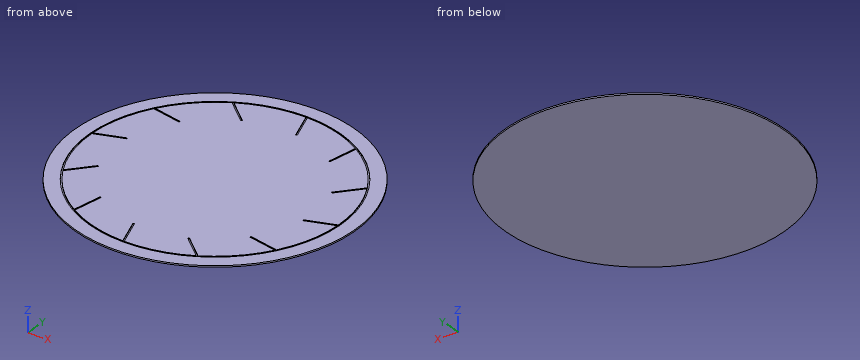
from build123d import *

# Parameters (mm, degrees)
SKETCH1_R           = 254
BOSS_EXTRUDE1_DEPTH = 2.54
SKETCH2_R           = 228.6
SKETCH2_R_2         = 226.06
CUT_EXTRUDE1_DEPTH  = 1.27
CUT_EXTRUDE2_DEPTH  = 1.27


with BuildPart() as part:
    # Sketch1 → Boss-Extrude1 (new body)
    with BuildSketch(Plane.XY):
        Circle(SKETCH1_R)
    extrude(amount=BOSS_EXTRUDE1_DEPTH)

    # Sketch2 → Cut-Extrude1 (cut)
    with BuildSketch(Plane.XY.offset(2.54)):
        Circle(SKETCH2_R)
        Circle(SKETCH2_R_2, mode=Mode.SUBTRACT)
    extrude(amount=-CUT_EXTRUDE1_DEPTH, mode=Mode.SUBTRACT)

    # Sketch4 → Cut-Extrude2 (cut)
    with BuildSketch(Plane.XY.offset(2.54)):
        with BuildLine():
            Line((-226.06, 0), (-175.26, 18.489687901))
            Line((-175.26, 18.489687901), (-176.128731164, 20.876507158))
            Line((-176.128731164, 20.876507158), (-226.043768674, 2.708919262))
            ThreePointArc((-226.043768674, 2.708919262), (-226.055942132, 1.354483944), (-226.06, 0))
        make_face()
        with BuildLine():
            Line((-195.77370278, 113.03), (-142.534768317, 103.64253943))
            Line((-142.534768317, 103.64253943), (-142.093701946, 106.143951123))
            Line((-142.093701946, 106.143951123), (-194.405186408, 115.367877234))
            ThreePointArc((-194.405186408, 115.367877234), (-195.092946591, 114.200988571), (-195.77370278, 113.03))
        make_face()
        with BuildLine():
            Line((-113.03, 195.77370278), (-71.61746057, 161.024456218))
            Line((-71.61746057, 161.024456218), (-69.984780041, 162.970209103))
            Line((-69.984780041, 162.970209103), (-110.67589144, 197.11410567))
            ThreePointArc((-110.67589144, 197.11410567), (-111.854953561, 196.447430535), (-113.03, 195.77370278))
        make_face()
        with BuildLine():
            Line((0, 226.06), (18.489687901, 175.26))
            Line((18.489687901, 175.26), (20.876507158, 176.128731164))
            Line((20.876507158, 176.128731164), (2.708919262, 226.043768674))
            ThreePointArc((2.708919262, 226.043768674), (1.354483944, 226.055942132), (0, 226.06))
        make_face()
        with BuildLine():
            Line((113.03, 195.77370278), (103.64253943, 142.534768317))
            Line((103.64253943, 142.534768317), (106.143951123, 142.093701946))
            Line((106.143951123, 142.093701946), (115.367877234, 194.405186408))
            ThreePointArc((115.367877234, 194.405186408), (114.200988571, 195.092946591), (113.03, 195.77370278))
        make_face()
        with BuildLine():
            Line((195.77370278, 113.03), (161.024456218, 71.61746057))
            Line((161.024456218, 71.61746057), (162.970209103, 69.984780041))
            Line((162.970209103, 69.984780041), (197.11410567, 110.67589144))
            ThreePointArc((197.11410567, 110.67589144), (196.447430535, 111.854953561), (195.77370278, 113.03))
        make_face()
        with BuildLine():
            Line((226.06, 0), (175.26, -18.489687901))
            Line((175.26, -18.489687901), (176.128731164, -20.876507158))
            Line((176.128731164, -20.876507158), (226.043768674, -2.708919262))
            ThreePointArc((226.043768674, -2.708919262), (226.055942132, -1.354483944), (226.06, 0))
        make_face()
        with BuildLine():
            Line((195.77370278, -113.03), (142.534768317, -103.64253943))
            Line((142.534768317, -103.64253943), (142.093701946, -106.143951123))
            Line((142.093701946, -106.143951123), (194.405186408, -115.367877234))
            ThreePointArc((194.405186408, -115.367877234), (195.092946591, -114.200988571), (195.77370278, -113.03))
        make_face()
        with BuildLine():
            Line((113.03, -195.77370278), (71.61746057, -161.024456218))
            Line((71.61746057, -161.024456218), (69.984780041, -162.970209103))
            Line((69.984780041, -162.970209103), (110.67589144, -197.11410567))
            ThreePointArc((110.67589144, -197.11410567), (111.854953561, -196.447430535), (113.03, -195.77370278))
        make_face()
        with BuildLine():
            Line((0, -226.06), (-18.489687901, -175.26))
            Line((-18.489687901, -175.26), (-20.876507158, -176.128731164))
            Line((-20.876507158, -176.128731164), (-2.708919262, -226.043768674))
            ThreePointArc((-2.708919262, -226.043768674), (-1.354483944, -226.055942132), (0, -226.06))
        make_face()
        with BuildLine():
            Line((-113.03, -195.77370278), (-103.64253943, -142.534768317))
            Line((-103.64253943, -142.534768317), (-106.143951123, -142.093701946))
            Line((-106.143951123, -142.093701946), (-115.367877234, -194.405186408))
            ThreePointArc((-115.367877234, -194.405186408), (-114.200988571, -195.092946591), (-113.03, -195.77370278))
        make_face()
        with BuildLine():
            Line((-195.77370278, -113.03), (-161.024456218, -71.61746057))
            Line((-161.024456218, -71.61746057), (-162.970209103, -69.984780041))
            Line((-162.970209103, -69.984780041), (-197.11410567, -110.67589144))
            ThreePointArc((-197.11410567, -110.67589144), (-196.447430535, -111.854953561), (-195.77370278, -113.03))
        make_face()
    extrude(amount=-CUT_EXTRUDE2_DEPTH, mode=Mode.SUBTRACT)


solid = part.part
Geometry: final body of the model. Coordinates: model frame, mm. Give positions to 0.01 mm unless a question says otherwise; leave off trailing zeros. Loops run counter-clockwise (first coordinate to the right, second up) from the corner with the lowest first, then second, coordinate; pieces in that order, holes last. Notation, with made-up numbers: (-16.5, 53) - (33.5, 53) arc R20 cw to (33.5, 68) - close; hole circle Ø1 at (-17.75, -39.5). An arc over 180 degrees is marked (long way). One line per question, with ' | ' between items. Start each with the question number.
(1) Section query A-A on z = 1.85. Count the separate pieces of the cut face and the enclosed holes in it, then the cut area to 3 significant figures.
(2) Section query B-B on y = -52. Return loops of the section in (x, z).
(3) Section query C-C on x = 125. Return loops of the section in (y, z), then the cut area to 3 significant figures.
(4) Section query D-D on x = -87.5. Return loops of the section in (y, z), then the cut area to 3 significant figures.
(5) Ray query, line 1 (X direction, y = 43, z = 2.1); line 2 (X direction, y = -38.5, z = 2); line 3 (X direction, y = 157.5, z = 1.7). Return the intervals inside material, ascending. Write a range as from..to.
The answers:
1) separate pieces: 2 | enclosed holes: 1 | area: 197,000 mm2
2) outline: (-248.62, 0) - (248.62, 0) - (248.62, 2.54) - (222.61, 2.54) - (222.61, 1.27) - (220, 1.27) - (220, 2.54) - (-220, 2.54) - (-220, 1.27) - (-222.61, 1.27) - (-222.61, 2.54) - (-248.62, 2.54) - close
3) outline: (-221.11, 0) - (221.11, 0) - (221.11, 2.54) - (191.4, 2.54) - (191.4, 1.27) - (188.36, 1.27) - (188.36, 2.54) - (-188.36, 2.54) - (-188.36, 1.27) - (-191.4, 1.27) - (-191.4, 2.54) - (-221.11, 2.54) - close | area: 1,120 mm2
4) outline: (-238.45, 0) - (238.45, 0) - (238.45, 2.54) - (211.19, 2.54) - (211.19, 1.27) - (208.44, 1.27) - (208.44, 2.54) - (177.67, 2.54) - (177.67, 1.27) - (174.35, 1.27) - (174.35, 2.54) - (-208.44, 2.54) - (-208.44, 1.27) - (-211.19, 1.27) - (-211.19, 2.54) - (-238.45, 2.54) - close | area: 1,200 mm2
5) line 1: -250.33..-224.52, -221.93..221.93, 224.52..250.33 | line 2: -251.07..-225.33, -222.76..222.76, 225.33..251.07 | line 3: -199.27..-165.69, -162.16..106.28, 108.86..162.16, 165.69..199.27
